Input: part model. Units: mm. Frame: model coordinates. Face numbers are marked on the shaded views. A direction names the side the tool comes from. Round coordinates to 2 decimals unless told otherwise and drop trailing zeros. Loops run counter-clockwise (first coordinate to the right, second up) from the corner with the lowest first, then second, coordinate; pieces in that order, holes last. Notation, with made-up numbers: (43.25, 52.5) -> (91.25, 52.5) arc R18 cw to (91.25, 61.5) -> close; hole circle Ø5 at (87, 40). An arc over 180 degrees is marked (long way). Answer as a JSON object with one key per item and string values. Group by question number.
Item 1: Draft query along Y for the marked faces 6, 7 and 8. Return one class per face: released by +Y, released by -Y, zero draft, split by the parting line, or undercut.
Item 2: Pin query (flat end, axial travel): pin 1 (1.5 mm diameter, centred on x = 9.5, y = 8.5, fed in from -Z); pin 2 (14 mm diameter, centred on x = 22.5, y = 36, fed in from +Z); pin 3 (3.5 mm diameter, centred on x = 3.5, z = 16, fed in from +Y). Return the tip coordinate at first contact, or that it passes through.
Item 3: Set-up query: the marked faces 1, 2, 3, 4 and 5. Return all of +Z, -Z, +X, -X, +Y, -Y with unobstructed straight access to the full face (end or side cutting, diameter ignored); none if empty.
Item 4: Section query C-C on x = 12.7. Count the separate pieces of the cut face and the enclosed holes in it, and give its area (3 significant figures).
Item 5: Section query A-A on y = 38.1. Return loops of the section in (x, z) (3 decimals), and give its area (3 significant figures).
Item 6: Section query B-B on x = 25.4. Return loops of the section in (y, z) (3 decimals).
Item 7: Material intervals for line 1 (Y direction, x = 44.5, z = 9.25); line 2 (X direction, y = 38.1, z = 0.45) (3 decimals), sorted ascending. Write a range as [from, to].
from build123d import *

# Parameters (mm, degrees)
SKETCH1_W          = 50.8
SKETCH1_H          = 50.8
MAIN_BODY_DEPTH    = 18.288
SKETCH2_W          = 7.112
SKETCH2_H          = 28.448
FRONT_CUT_DEPTH    = 75.133197314
SHELL1_T           = -2.032
SKETCH3_R          = 13.5001
CENTER_HOLE_DEPTH  = 75.133197314
FILL060_VERT_R     = 1.524
FILL060_TB_R       = 1.524
CHAM025_SIZE       = 0.635
KEYED_HOLE_1_DEPTH = 60.460200948


with BuildPart() as part:
    # Sketch1 → main body (new body)
    with BuildSketch(Plane.XY):
        with Locations((25.4, 25.4)):
            Rectangle(SKETCH1_W, SKETCH1_H)
    extrude(amount=MAIN_BODY_DEPTH)

    # Sketch2 → front cut (cut, through all)
    with BuildSketch(Plane(origin=(50.8, 0, 0), x_dir=(0, 0, -1), z_dir=(1, 0, 0))):
        with Locations((-14.732, 36.576)):
            Rectangle(SKETCH2_W, SKETCH2_H)
    extrude(amount=-FRONT_CUT_DEPTH, mode=Mode.SUBTRACT)

    # Shell1
    shell1_openings = [part.faces().sort_by_distance(p)[0] for p in [
        (25.4, 36.576, 11.176),
        (25.4, 22.352, 14.732),
    ]]
    offset(amount=SHELL1_T, openings=shell1_openings, kind=Kind.INTERSECTION)

    # Sketch3 → center hole (cut, through all)
    with BuildSketch(Plane.XY):
        with Locations((25.4, 22.352)):
            Circle(SKETCH3_R)
    extrude(amount=CENTER_HOLE_DEPTH, mode=Mode.SUBTRACT)

    # fill060.vert
    fill060_vert_edges = [part.edges().sort_by_distance(p)[0] for p in [
        (2.032, 12.192, 16.256),
        (48.768, 12.192, 16.256),
        (2.032, 25.4, 2.032),
        (48.768, 25.4, 2.032),
    ]]
    fillet(fill060_vert_edges, radius=FILL060_VERT_R)

    # fill060.tb
    fill060_tb_edges = [part.edges().sort_by_distance(p)[0] for p in [
        (2.032, 48.768, 7.366),
        (48.768, 48.768, 7.366),
        (25.4, 2.032, 16.256),
        (25.4, 2.032, 2.032),
        (2.032, 2.032, 9.144),
        (48.768, 2.032, 9.144),
        (2.478369265, 2.032, 15.809630735),
        (2.478369265, 2.032, 2.478369265),
        (48.321630735, 2.032, 2.478369265),
        (48.321630735, 2.032, 15.809630735),
        (25.4, 48.768, 2.032),
        (2.478369265, 48.768, 2.478369265),
        (48.321630735, 48.768, 2.478369265),
    ]]
    fillet(fill060_tb_edges, radius=FILL060_TB_R)

    # cham025
    cham025_edges = [part.edges().sort_by_distance(p)[0] for p in [
        (11.8999, 22.352, 0),
        (25.4, 8.8519, 18.288),
    ]]
    chamfer(cham025_edges, length=CHAM025_SIZE)

    # Sketch6 → Keyed Hole 1 (cut, through all)
    with BuildSketch(Plane(origin=(10.255789697, 39.461773448, 0), x_dir=(-1, 0, 0), z_dir=(0, 0, -1))):
        with BuildLine():
            Line((0.603789697, -0.472773448), (2.000789697, -0.472773448))
            Line((2.000789697, -0.472773448), (2.000789697, -2.250773448))
            Line((2.000789697, -2.250773448), (0.603789697, -2.250773448))
            ThreePointArc((0.603789697, -2.250773448), (-5.619210303, -1.361773448), (0.603789697, -0.472773448))
        make_face()
    keyed_hole_1 = extrude(amount=-KEYED_HOLE_1_DEPTH, mode=Mode.SUBTRACT)

    # Mirror 1: Keyed Hole 1 across plane
    add(keyed_hole_1.mirror(Plane(origin=(25.4, 0, 0), x_dir=(0, 0, 1), z_dir=(1, 0, 0))), mode=Mode.SUBTRACT)


solid = part.part
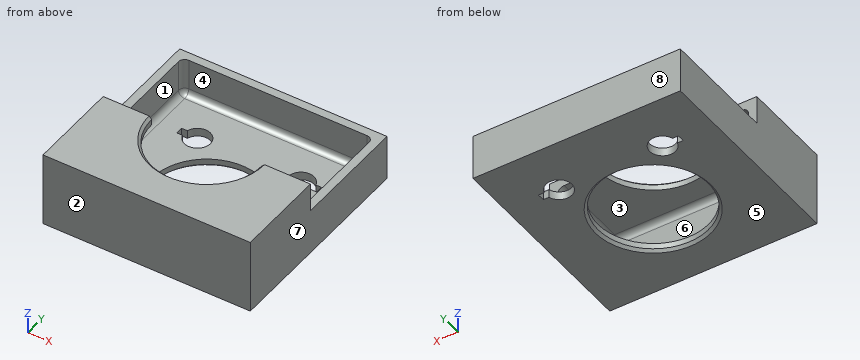
Solved:
{
 "1": {"face 6": "undercut", "face 7": "zero draft", "face 8": "released by +Y"},
 "2": {"pin 1": "z = 0", "pin 2": "z = 2.03", "pin 3": "y = 22.35"},
 "3": {"face 1": "none", "face 2": "+Z, -Z, +X, -X, -Y", "face 3": "+Y", "face 4": "+Z", "face 5": "-Z, +X, -X, +Y, -Y"},
 "4": {"separate pieces": "3", "enclosed holes": "0", "area": "155 mm²"},
 "5": {"outline": "(0, 0) -> (8.255, 0) -> (8.255, 2.032) -> (3.556, 2.032) arc R1.524 cw to (2.032, 3.556) -> (2.032, 11.176) -> (0, 11.176) -> close; (15.875, 0) -> (34.925, 0) -> (34.925, 2.032) -> (15.875, 2.032) -> close; (42.545, 0) -> (50.8, 0) -> (50.8, 11.176) -> (48.768, 11.176) -> (48.768, 3.556) arc R1.524 cw to (47.244, 2.032) -> (42.545, 2.032) -> close", "area": "110 mm²"},
 "6": {"outline": "(0, 0) -> (8.217, 0) -> (8.852, 0.635) -> (8.852, 2.032) -> (3.556, 2.032) arc R1.524 cw to (2.032, 3.556) -> (2.032, 14.732) arc R1.524 cw to (3.556, 16.256) -> (8.852, 16.256) -> (8.852, 17.653) -> (8.217, 18.288) -> (0, 18.288) -> close; (35.852, 0.635) -> (36.487, 0) -> (50.8, 0) -> (50.8, 11.176) -> (48.768, 11.176) -> (48.768, 3.556) arc R1.524 cw to (47.244, 2.032) -> (35.852, 2.032) -> close"},
 "7": {"line 1": "[0, 2.03], [48.77, 50.8]", "line 2": "[0, 8.255], [15.875, 34.925], [42.545, 50.8]"}
}
